Read the model definition and answer for the solid it produces. Units are mm, in the model's axes. A direction names the side the tool comes from. Round coordinates to 2 decimals unless told otherwise and drop trailing zeros. Order: outer loops, then holes, each group sorted by start corner. A loop starts at its lowest first (then second) coordinate and runs counter-clockwise, first axis right, second up. Notation, with made-up numbers: (43.25, -20) -> (87.25, -20) arc R9 ccw to (87.25, -9) -> close; hole circle Ø9 at (64, 16). An arc over 180 degrees is marked (long way). Answer as a JSON object with one key per item and string values. Group by question number.
Item 1: Consider probe 1 along Y at (x, z) = (10, 25.4); probe 2 along Y at (x, z) = (3, 25); probe 3 along X at (y, z) = (-74, 10). Determine where each line is inside the solid, lowest interval first. Write a range as from..to.
Item 2: Given P1, Ø21.5, axis at x = 127, z = 20.5, coming from the -Y side; P2, Ø5, axis at y = -31.75, z = 25.4, coming from the +X side; P3, Ø8, axis at y = -54.5, z = 23, coming from the +X side, each flat-ended and moving along its own axis, determine where each tip first touches the part or whether it passes through.
Item 3: Section B-B, the plane x = 130.5 is taken. Write down the section's boundary in (y, z), plus the area to 3 significant figures.
Item 4: Section C-C, the plane x = 82.5 is taken. Write down the section's boundary in (y, z).
Item 5: Section A-A, the plane z = 25.4 is taken. Write down the section's boundary in (x, y), plus the area to 3 significant figures.
Item 6: For faces 5 (the flat face through (6.35, -33, 23)), 6 (the flat face through (32, -38, 43.18)), 7 (the flat face through (63, -26, 50.8)), determine the directions among +Z, -Z, +X, -X, +Y, -Y from which every point of the face is accessible in a straight line to the end or side of a thin tool.
Item 7: The mould has two halves that part along Y. Classify faces 1 (the flat face through (0, -53, 25)), 2 (the flat face through (90, 0, 25)), 3 (the cylindrical face through (12.789, -30.319, 20.857)), 4 (the flat face through (9, -107.95, 25)): pulls with the +Y half, pulls with the -Y half, needs draft (parallel to the pull), parting line crosses it, or undercut.
from build123d import *

# Parameters (mm, degrees)
BOSS_EXTRUDE1_DEPTH                                 = 50.8
F_8_CLEARANCE_HOLE1_D                               = 4.4958
CBORE_FOR_8_BINDING_HEAD_MACHINE_SCREW1_D           = 4.4958
CBORE_FOR_8_BINDING_HEAD_MACHINE_SCREW1_CBORE_D     = 9.525
CBORE_FOR_8_BINDING_HEAD_MACHINE_SCREW1_CBORE_DEPTH = 12.7
BOSS_EXTRUDE2_DEPTH                                 = 7.62
CUT_EXTRUDE1_DEPTH                                  = 7.62


with BuildPart() as part:
    # Sketch1 → Boss-Extrude1 (new body)
    with BuildSketch(Plane.XY):
        Polygon((0, 0), (0, -107.95), (19.05, -107.95), (19.05, -25.4), (177.8, -25.4), (177.8, 0), align=None)
    extrude(amount=BOSS_EXTRUDE1_DEPTH)

    # #8 Clearance Hole1 (through all)
    with Locations(Plane.ZY):
        with Locations((25.4, -31.75), (25.4, -88.9)):
            Hole(F_8_CLEARANCE_HOLE1_D / 2)

    # CBORE for #8 Binding Head Machine Screw1 (through all)
    with Locations(Plane(origin=(19.05, 0, 0), x_dir=(0, 0, -1), z_dir=(1, 0, 0))):
        with Locations((-25.4, -31.75), (-25.4, -88.9)):
            CounterBoreHole(CBORE_FOR_8_BINDING_HEAD_MACHINE_SCREW1_D / 2, CBORE_FOR_8_BINDING_HEAD_MACHINE_SCREW1_CBORE_D / 2, CBORE_FOR_8_BINDING_HEAD_MACHINE_SCREW1_CBORE_DEPTH)

    # Sketch7 → Boss-Extrude2 (add)
    with BuildSketch(Plane.XY.offset(50.8)):
        with BuildLine():
            Line((19.05, -107.95), (19.05, -25.4))
            Line((19.05, -25.4), (177.8, -25.4))
            ThreePointArc((177.8, -25.4), (91.430997476, -53.224995146), (19.05, -107.95))
        make_face()
    boss_extrude2 = extrude(amount=-BOSS_EXTRUDE2_DEPTH)

    # Mirror1: Boss-Extrude2 across plane
    add(boss_extrude2.mirror(Plane(origin=(0, 0, 25.4), x_dir=(1, 0, 0), z_dir=(0, 0, -1))))

    # Sketch8 → Cut-Extrude1 (cut)
    with BuildSketch(Plane.XY.offset(50.8)):
        with BuildLine():
            Line((177.8, -25.4), (80.273648103, -25.4))
            add(Edge.make_bspline(
                [(80.273648103, -25.4), (36.871479527, -25.4), (15.065136677, -63.527261514), (19.05, -107.95)],
                knots=[0, 0, 0, 0, 1, 1, 1, 1], degree=3))
            Line((19.05, -107.95), (177.8, -25.4))
        make_face()
    extrude(amount=-CUT_EXTRUDE1_DEPTH, mode=Mode.SUBTRACT)


solid = part.part
Values found:
{
 "1": {"probe 1": "-107.95..-93.66, -84.14..-36.51, -26.99..0", "probe 2": "-107.95..-91.11, -86.69..-33.96, -29.54..0", "probe 3": "0..19.05"},
 "2": {"P1": "y = -25.4", "P2": "x = 6.35", "P3": "x = 19.05"},
 "3": {"outline": "(-36.65, 0) -> (0, 0) -> (0, 50.8) -> (-25.4, 50.8) -> (-25.4, 7.62) -> (-36.65, 7.62) -> close", "area": "1,380 mm2"},
 "4": {"outline": "(-58.08, 0) -> (0, 0) -> (0, 50.8) -> (-25.4, 50.8) -> (-25.4, 7.62) -> (-58.08, 7.62) -> close"},
 "5": {"outline": "(0, -107.95) -> (19.05, -107.95) -> (19.05, -93.66) -> (6.35, -93.66) -> (6.35, -91.15) -> (0, -91.15) -> close; (0, -86.65) -> (6.35, -86.65) -> (6.35, -84.14) -> (19.05, -84.14) -> (19.05, -36.51) -> (6.35, -36.51) -> (6.35, -34) -> (0, -34) -> close; (0, -29.5) -> (6.35, -29.5) -> (6.35, -26.99) -> (19.05, -26.99) -> (19.05, -25.4) -> (177.8, -25.4) -> (177.8, 0) -> (0, 0) -> close", "area": "5,790 mm2"},
 "6": {"face 5": "+X", "face 6": "+X, -Y", "face 7": "+Z, +X, -X, +Y, -Y"},
 "7": {"face 1": "needs draft", "face 2": "pulls with the +Y half", "face 3": "undercut", "face 4": "pulls with the -Y half"}
}
